```python
from build123d import *

# Parameters (mm, degrees)
F0_W     = 10
F0_H     = 5
F1_DEPTH = 2
F2_W     = 10
F2_H     = 5
F3_DEPTH = 20
F4_W     = 10
F4_H     = 5
F5_DEPTH = 2


with BuildPart() as f1:
    # F0 (on Top) → F1 (new body)
    with BuildSketch(Plane.XY):
        Polygon((4.999269, -35), (4.999269, -15), (-4.999269, -15), (-5.000731, -15), (-5.000731, -35), align=None)
        Polygon((-4.999269, -15), (4.999269, -15), (4.999269, 10), (-5.000731, 10), (-5.000731, -15), align=None)
        with Locations((-0.000731, 12.5)):
            Rectangle(F0_W, F0_H)
    extrude(amount=F1_DEPTH)

    # F2 (on face) → F3 (join)
    with BuildSketch(Plane.XY.offset(2)):
        with Locations((-0.000731, 12.5)):
            Rectangle(F2_W, F2_H)
    extrude(amount=F3_DEPTH)

    # F4 (on face) → F5 (join)
    with BuildSketch(Plane.XY.offset(22)):
        Polygon((-5.000731, 10), (-5.000731, 15), (-25, 15), (-25, -15), (-5.000731, -15), align=None)
        Polygon((4.999269, -15), (4.999269, 10), (-5.000731, 10), (-5.000731, -15), (-4.999269, -15), align=None)
        with Locations((-0.000731, 12.5)):
            Rectangle(F4_W, F4_H)
        Polygon((25, -15), (25, 15), (4.999269, 15), (4.999269, 10), (4.999269, -15), align=None)
    extrude(amount=F5_DEPTH)


solid = f1.part
```
Can you work these out from the model? Positions are in its coordinate system, mm. A direction names the side the tool comes from. Coordinates: 2 decimals unless noted, no trailing zeros. Order: outer loops, then holes, each group sorted by start corner. A loop starts at its lowest first (then second) coordinate and runs counter-clockwise, first axis right, second up. Notation, with made-up numbers: (89.25, 76) - (147.25, 76) arc R18 ccw to (147.25, 104) - close; hole circle Ø6 at (81.25, 80.25). An arc over 180 degrees is marked (long way). Answer in a Markdown table with one row per item.
1. If we mould it in two halves opening along Z, with no side actions, what happens to faces 1 (the flat face through (0, -10, 0)), 2 (the flat face through (0, 15, 15)), 3 (the flat face through (0, 10, 12)), 4 (the flat face through (0, -12, 2))? For each: pulls with the +Z half, pulls with the -Z half, needs draft (parallel to the pull), parting line crosses it, or undercut.
Reply:
| item | result |
|---|---|
| face 1 | pulls with the -Z half |
| face 2 | needs draft |
| face 3 | undercut |
| face 4 | undercut |
2. For faces 5 (the flat face through (-5.001, 1, 1)), 6 (the flat face through (0, 0, 24)), 7 (the flat face through (4.999, 1, 1)), which set-ups out of +Z, -Z, +X, -X, +Y, -Y let a thin tool reach every point of the face, with its end or its side?
Reply:
| item | result |
|---|---|
| face 5 | -Z, -X, +Y, -Y |
| face 6 | +Z, +X, -X, +Y, -Y |
| face 7 | -Z, +X, +Y, -Y |
3. Suppose I cut it at C-C (z = 7). Please give me the cut outline in (x, y).
Reply:
| item | result |
|---|---|
| outline | (-5, 10) - (5, 10) - (5, 15) - (-5, 15) - close |
4. Suppose I cut it at D-D (y = -19). Please give me the cut outline in (x, z).
Reply:
| item | result |
|---|---|
| outline | (-5, 0) - (5, 0) - (5, 2) - (-5, 2) - close |
5. For pin 1 (1 mm diameter, centred on x = 0, y = -8.5, fed in from -Z); pin 2 (11 mm diameter, centred on x = -2, z = 11.5, fed in from -Y); pin 3 (1.6 mm diameter, centred on x = 9.5, z = 23.5, fed in from -Y); pin 4 (8 mm diameter, centred on y = 7, z = 4, fed in from -X), each with a flat end and sliding along its axis, tell me the tip position at first contact or that it passes through.
Reply:
| item | result |
|---|---|
| pin 1 | stops at z = 0 |
| pin 2 | stops at y = 10 |
| pin 3 | stops at y = -15 |
| pin 4 | stops at x = -5 |
6. If I drill on line 1 along Z through (x, y) = (-2, -11.5); line 2 along Z through (x, y) = (-8.5, -12); line 3 along Y through (x, z) = (-2, 11.75), over which ranges is the centre line in solid material (lowest first)?
Reply:
| item | result |
|---|---|
| line 1 | z = 0 to 2, 22 to 24 |
| line 2 | z = 22 to 24 |
| line 3 | y = 10 to 15 |
7. Suppose I cut it at A-A (y = 0.5). Please give me the cut outline in (x, z), and give its area (3 significant figures).
Reply:
| item | result |
|---|---|
| outline | (-25, 22) - (25, 22) - (25, 24) - (-25, 24) - close; (-5, 0) - (5, 0) - (5, 2) - (-5, 2) - close |
| area | 120 mm^2 |
8. Suppose I cut it at B-B (x = -2). Please give me the cut outline in (y, z), and give its area (3 significant figures).
Reply:
| item | result |
|---|---|
| outline | (-35, 0) - (15, 0) - (15, 24) - (-15, 24) - (-15, 22) - (10, 22) - (10, 2) - (-35, 2) - close |
| area | 260 mm^2 |
